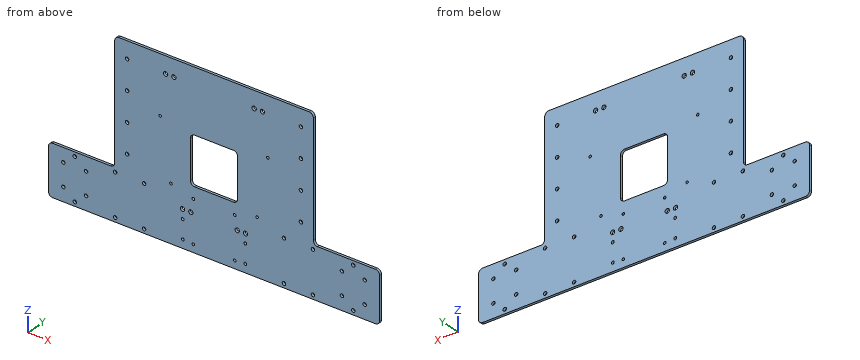
```python
from build123d import *

# Parameters (mm, degrees)
SKETCH_1_R          = 1.6
SKETCH_1_W          = 57
SKETCH_1_H          = 57
EXTRUDE_1451_DEPTH  = 3
SKETCH_2_R          = 2.05
SKETCH_2_R_2        = 2.1
CUT_EXTRUDE_1_DEPTH = 287.415781688
FILLET_1_R          = 5
SKETCH_3_R          = 2.1
SKETCH_3_R_2        = 1.55
SKETCH_3_R_3        = 2.6
CUT_EXTRUDE_2_DEPTH = 287.415781688
SKETCH_4_R          = 1.75
CUT_EXTRUDE_3_DEPTH = 10


with BuildPart() as part:
    # 草图1 → Extrude 1451 (new body)
    # profile 1 of 2: a face of its own
    with BuildSketch(Plane(origin=(0, 0, 0), x_dir=(1, 0, 0), z_dir=(0, 1, 0))):
        with BuildLine():
            Line((-200, 0), (-200, -60))
            Line((-200, -60), (-120, -60))
            Line((-120, -60), (-26.385640646, -60))
            ThreePointArc((-26.385640646, -60), (-25.414110472, -57.654518678), (-23.4, -59.2))
            ThreePointArc((-23.4, -59.2), (-23.454518678, -59.614110472), (-23.614359354, -60))
            Line((-23.614359354, -60), (23.614359354, -60))
            ThreePointArc((23.614359354, -60), (24.585889528, -57.654518678), (26.6, -59.2))
            ThreePointArc((26.6, -59.2), (26.545481322, -59.614110472), (26.385640646, -60))
            Line((26.385640646, -60), (120, -60))
            Line((120, -60), (200, -60))
            Line((200, -60), (200, 0))
            Line((200, 0), (-200, 0))
        make_face()
        with Locations(Location((-25, -9.2, 0), (0, 0, 270))):
            Circle(SKETCH_1_R, mode=Mode.SUBTRACT)
        with Locations(Location((25, -9.2, 0), (0, 0, 270))):
            Circle(SKETCH_1_R, mode=Mode.SUBTRACT)
    # profile 2 of 2: a face of its own
    with BuildSketch(Plane(origin=(0, 0, 0), x_dir=(1, 0, 0), z_dir=(0, 1, 0))):
        with BuildLine():
            Line((-26.385640646, -60), (-120, -60))
            Line((-120, -60), (-120, -205))
            Line((-120, -205), (120, -205))
            Line((120, -205), (120, -60))
            Line((120, -60), (26.385640646, -60))
            ThreePointArc((26.385640646, -60), (25, -60.8), (23.614359354, -60))
            Line((23.614359354, -60), (-23.614359354, -60))
            ThreePointArc((-23.614359354, -60), (-25, -60.8), (-26.385640646, -60))
        make_face()
        with Locations((0, -101.5)):
            Rectangle(SKETCH_1_W, SKETCH_1_H, mode=Mode.SUBTRACT)
    extrude(amount=EXTRUDE_1451_DEPTH)

    # 草图2 → 切除-拉伸1 (cut, through all)
    with BuildSketch(Plane(origin=(0, 3, 0), x_dir=(1, 0, 0), z_dir=(0, 1, 0))):
        with Locations(Location((-182, -16.5, 0), (0, 0, 270))):
            Circle(SKETCH_2_R)
        with Locations(Location((-182, -43.5, 0), (0, 0, 270))):
            Circle(SKETCH_2_R)
        with Locations(Location((-154.5, -16.5, 0), (0, 0, 270))):
            Circle(SKETCH_2_R)
        with Locations(Location((-154.5, -43.5, 0), (0, 0, 90))):
            Circle(SKETCH_2_R)
        with Locations(Location((-84.5, -5, 0), (0, 0, 270))):
            Circle(SKETCH_2_R_2)
        with Locations(Location((-119.5, -5, 0), (0, 0, 270))):
            Circle(SKETCH_2_R_2)
        with Locations(Location((-84.5, -55, 0), (0, 0, 90))):
            Circle(SKETCH_2_R_2)
        with Locations(Location((-119.5, -55, 0), (0, 0, 90))):
            Circle(SKETCH_2_R_2)
        with Locations(Location((-168.25, -5, 0), (0, 0, 270))):
            Circle(SKETCH_2_R_2)
        with Locations(Location((-168.25, -55, 0), (0, 0, 90))):
            Circle(SKETCH_2_R_2)
        with Locations(Location((168.25, -55, 0), (0, 0, 270))):
            Circle(SKETCH_2_R_2)
        with Locations(Location((168.25, -5, 0), (0, 0, 90))):
            Circle(SKETCH_2_R_2)
        with Locations(Location((119.5, -55, 0), (0, 0, 270))):
            Circle(SKETCH_2_R_2)
        with Locations(Location((84.5, -55, 0), (0, 0, 270))):
            Circle(SKETCH_2_R_2)
        with Locations(Location((119.5, -5, 0), (0, 0, 90))):
            Circle(SKETCH_2_R_2)
        with Locations(Location((84.5, -5, 0), (0, 0, 90))):
            Circle(SKETCH_2_R_2)
        with Locations(Location((154.5, -43.5, 0), (0, 0, 270))):
            Circle(SKETCH_2_R)
        with Locations(Location((154.5, -16.5, 0), (0, 0, 90))):
            Circle(SKETCH_2_R)
        with Locations(Location((182, -43.5, 0), (0, 0, 90))):
            Circle(SKETCH_2_R)
        with Locations(Location((182, -16.5, 0), (0, 0, 90))):
            Circle(SKETCH_2_R)
    extrude(amount=-CUT_EXTRUDE_1_DEPTH, mode=Mode.SUBTRACT)

    # 圆角1
    fillet_1_edges = [part.edges().sort_by_distance(p)[0] for p in [
        (-28.5, 1.5, 73),
        (-28.5, 1.5, 130),
        (28.5, 1.5, 130),
        (28.5, 1.5, 73),
        (120, 1.5, 205),
        (-120, 1.5, 205),
        (-120, 1.5, 60),
        (-200, 1.5, 60),
        (-200, 1.5, 0),
        (200, 1.5, 0),
        (200, 1.5, 60),
        (120, 1.5, 60),
    ]]
    fillet(fillet_1_edges, radius=FILLET_1_R)

    # 草图3 → 切除-拉伸2 (cut, through all)
    with BuildSketch(Plane(origin=(0, 3, 0), x_dir=(1, 0, 0), z_dir=(0, 1, 0))):
        with Locations(Location((-105, -80, 0), (0, 0, 270))):
            Circle(SKETCH_3_R)
        with Locations(Location((-105, -115, 0), (0, 0, 270))):
            Circle(SKETCH_3_R)
        with Locations(Location((-105, -150, 0), (0, 0, 270))):
            Circle(SKETCH_3_R)
        with Locations(Location((-105, -185, 0), (0, 0, 270))):
            Circle(SKETCH_3_R)
        with Locations(Location((105, -185, 0), (0, 0, 90))):
            Circle(SKETCH_3_R)
        with Locations(Location((105, -150, 0), (0, 0, 90))):
            Circle(SKETCH_3_R)
        with Locations(Location((105, -115, 0), (0, 0, 90))):
            Circle(SKETCH_3_R)
        with Locations(Location((105, -80, 0), (0, 0, 90))):
            Circle(SKETCH_3_R)
        with Locations(Location((-52, -66.5, 0), (0, 0, 270))):
            Circle(SKETCH_3_R_2)
        with Locations(Location((-65, -136.5, 0), (0, 0, 270))):
            Circle(SKETCH_3_R_2)
        with Locations(Location((65, -136.5, 0), (0, 0, 90))):
            Circle(SKETCH_3_R_2)
        with Locations(Location((52, -66.5, 0), (0, 0, 90))):
            Circle(SKETCH_3_R_2)
        with Locations(Location((-38, -43.5, 0), (0, 0, 270))):
            Circle(SKETCH_3_R_3)
        with Locations(Location((-28, -43.5, 0), (0, 0, 270))):
            Circle(SKETCH_3_R_3)
        with Locations(Location((28, -43.5, 0), (0, 0, 90))):
            Circle(SKETCH_3_R_3)
        with Locations(Location((38, -43.5, 0), (0, 0, 90))):
            Circle(SKETCH_3_R_3)
        with Locations(Location((-58.5, -185, 0), (0, 0, 270))):
            Circle(SKETCH_3_R_3)
        with Locations(Location((-48.5, -185, 0), (0, 0, 270))):
            Circle(SKETCH_3_R_3)
        with Locations(Location((48.5, -185, 0), (0, 0, 90))):
            Circle(SKETCH_3_R_3)
        with Locations(Location((58.5, -185, 0), (0, 0, 90))):
            Circle(SKETCH_3_R_3)
    extrude(amount=-CUT_EXTRUDE_2_DEPTH, mode=Mode.SUBTRACT)

    # 草图4 → 切除-拉伸3 (cut)
    with BuildSketch(Plane(origin=(0, 3, 0), x_dir=(1, 0, 0), z_dir=(0, 1, 0))):
        with Locations(Location((-37.75, -10, 0), (0, 0, 270))):
            Circle(SKETCH_4_R)
        with Locations(Location((37.75, -10, 0), (0, 0, 270))):
            Circle(SKETCH_4_R)
        with Locations(Location((-37.75, -32.4, 0), (0, 0, 270))):
            Circle(SKETCH_4_R)
        with Locations(Location((37.75, -32.4, 0), (0, 0, 270))):
            Circle(SKETCH_4_R)
    extrude(amount=-CUT_EXTRUDE_3_DEPTH, mode=Mode.SUBTRACT)


solid = part.part
```
Could you check a few things on this model? Use its own coordinates, in mm. Coordinates: 2 decimals unless noted, no trailing zeros. Loops run counter-clockwise (first coordinate to the right, second up) from the corner with the lowest first, then second, coordinate; pieces in that order, holes last. Notation, with made-up numbers: M -40,21 L -30,21 A18 cw -30,43 Z; hole C 69,4 d10. An arc over 180 degrees is marked long. Put each result on its own line as item: value. Start each with the question number.
(1) I need wall thicknesses on line 1 (X direction, y = 1.6, z = 16.5); line 2 (X direction, y = 0.5, z = 32.5); line 3 (X direction, y = 1.3, z = 80). Which ranges of each line are inside material? Lowest first, please. Write a range as from..to.
(2) Suppose I cut it at B-B on x = -140. Please give me the cut outline in (y, z).
(3) Suppose I cut it at A-A on y = 2.45. Count the separate pieces of the cut face and the enclosed holes in it, then the cut area to 3 significant figures.
(4) Will this pin go through, and if not, where does the flat tip stop? P1, Ø1.5, axis at y = 1, z = 109, coming from the +X side.
Solutions:
1. line 1: x = -200..-184.05, -179.95..-156.55, -152.45..152.45, 156.55..179.95, 184.05..200
1. line 2: x = -200..-39.5, -36..36, 39.5..200
1. line 3: x = -120..-107.1, -102.9..-28.5, 28.5..102.9, 107.1..120
2. outline: M 0,0 L 3,0 L 3,60 L 0,60 Z
3. separate pieces: 1
3. enclosed holes: 49
3. area: 54,900 mm2
4. P1: stops at x = 120
